Autodesk Inventor part; units mm, degrees
ref_plane "Work Plane1" through (2.75, 0, 0) normal (0, -1, 0) x (1, 0, 0)
ref_plane "YZ Plane" through (0, 0, 0) normal (1, 0, 0) x (0, 1, 0)
ref_plane "XZ Plane" through (0, 0, 0) normal (0, 1, 0) x (-1, 0, 0)
sketch "Sketch1" plane through (0, 0, 0) normal (0, 0, 1) x (1, 0, 0)
  line L0 (50, 9) -> (50, 0)
  line L1 (-50, 0) -> (50, 0)
  line L2 (-70, 0) -> (70, 0)
  line L3 (0, 10.8) -> (0, -1.8)
  line L4 (-50, 9) -> (-50, 0)
  line L5 (0, 9) -> (0, 0) construction
  line L6 (-70, 0) -> (70, 0)
  line L7 (-50, 9) -> (50, 9)
  dimension "d13" = 18
  dimension "d87" = 100
  dimension "d88" = 50
revolve "Body" add sketch "Sketch1" angle 360 about axis through (-50, 0, 0) along (1, 0, 0)
thread "Thread1"
chamfer "Chamfer1" distance 1.035 angle 45 1 edges at (50, -9, 0) measured on face at (-16.6667, 8.8835, -1.4437)
chamfer "Chamfer2" distance 1.035 angle 45 1 edges at (-50, -9, 0) measured on face at (15.9767, 8.9708, -0.7242)
ref_plane "Work Plane1" through (2.75, 0, 0) normal (0, -1, 0) x (1, 0, 0)
equation "\"d13\" = NND"
equation "\"d87\" = NLG"
equation "\"d88\" = 0.5 * NLG"
equation "\"d1\" = GEL"
equation "\"d9\" = -0.5 * SPD + 0.5 * NND"
equation "\"d10\" = -0.5 * SPD + 0.5 * NND"
equation "\"d11\" = -0.5 * SPD + 0.5 * NND"
equation "\"d12\" = -0.5 * SPD + 0.5 * NND"
equation "\"NLG\" = 100"
equation "\"GEL\" = NLG"
equation "\"GAL\" = 0.61345 * PTC"
equation "\"SPD\" = 15.93"
equation "\"d0\" = NND"
equation "\"GUL\" = 0.61345 * PTC"
equation "\"NND\" = 18"
equation "\"GUL1\" = GUL"
equation "\"GAL1\" = GAL"
equation "\"d80\" = -GUL - GEL"
equation "\"d86\" = -GEL + GUL1"
equation "\"PTC\" = 1.5"
equation "\"THREADDIA\" = 18"
equation "\"TOA\" = 30deg"
equation "\"GD1\" = THREADDIA - 1.2269 * PTC"
properties part number "DIN 976-1 - M18 x 1.5 x 100 - B" material "Steel, Mild"
Geometry check sheet. Reference: the model listing, model coordinates, mm. Give positions to 0.01 mm unless a question says otherwise; leave off trailing zeros. Order: outer loops, then holes, each group sorted by start corner. A loop starts at its lowest first (then second) coordinate and runs counter-clockwise, first axis right, second up.
1. Scan lines: line 1 (Z direction, x = -15.5, y = 0.5); line 2 (Y direction, x = 12.5, z = 5). Record each from-to range of solid material in increasing order.
Completed:
line 1: z = -8.99 to 8.99
line 2: y = -7.48 to 7.48
2. Depth check by flat-ended pin: pin 1 (1.5 mm diameter, centred on x = -4.5, y = 4.5, fed in from +Z); pin 2 (1.5 mm diameter, centred on x = 29.5, z = -5, fed in from -Y); pin 3 (1.5 mm diameter, centred on x = -12, y = 2, fed in from +Z). Enter the tip coordinate at first touch or a pass-through.
Completed:
pin 1: stops at z = 8.18
pin 2: stops at y = -7.93
pin 3: stops at z = 8.91
3. Sectioned sample at A-A (x = -20). Record the boundary of the cut face in (y, z), then the cut area to 3 significant figures.
Completed:
outline: circle Ø18 at (0, 0)
area: 254 mm2
